```python
from build123d import *

# Parameters (mm, degrees)
ESQUISSE1_R             = 20
ESQUISSE1_R_2           = 8
BOSS_EXTRU_1_DEPTH      = 60
ESQUISSE2_W             = 40
ESQUISSE2_H             = 4.835178206
ESQUISSE2_W_2           = 44.689434038
ESQUISSE2_H_2           = 5.086258347
ENL_V_MAT_EXTRU_1_DEPTH = 60
TROU_TARAUD_M61_D       = 5
TROU_TARAUD_M61_DEPTH   = 13
TROU_TARAUD_M61_TIP     = 1.502151548
TROU_TARAUD_M62_D       = 5
TROU_TARAUD_M62_DEPTH   = 15
TROU_TARAUD_M62_TIP     = 1.502151548


with BuildPart() as part:
    # Esquisse1 → Boss.-Extru.1 (new body)
    with BuildSketch(Plane.XY):
        Circle(ESQUISSE1_R)
        Circle(ESQUISSE1_R_2, mode=Mode.SUBTRACT)
    extrude(amount=BOSS_EXTRU_1_DEPTH)

    # Esquisse2 → Enlèv. mat.-Extru.1 (cut)
    with BuildSketch(Plane.XY.offset(60)):
        with Locations((4.791370724, 19.417589103)):
            Rectangle(ESQUISSE2_W, ESQUISSE2_H)
        with Locations((-4.250423756, -19.543129173)):
            Rectangle(ESQUISSE2_W_2, ESQUISSE2_H_2)
    extrude(amount=-ENL_V_MAT_EXTRU_1_DEPTH, mode=Mode.SUBTRACT)

    # Trou taraudé M61
    with Locations(Plane(origin=(0, 17, 50), x_dir=(0, 0, 1), z_dir=(0, 1, 0))):
        with Locations((0, 0), (-40, 0)):
            Hole(TROU_TARAUD_M61_D / 2, depth=TROU_TARAUD_M61_DEPTH)
            with Locations((0, 0, -(TROU_TARAUD_M61_DEPTH + TROU_TARAUD_M61_TIP / 2))):  # 118° drill point
                Cone(0, TROU_TARAUD_M61_D / 2, TROU_TARAUD_M61_TIP, mode=Mode.SUBTRACT)

    # Trou taraudé M62
    with Locations(Plane(origin=(0, -17, 50), x_dir=(0, 0, -1), z_dir=(0, -1, 0))):
        with Locations((0, 0), (20, 0)):
            Hole(TROU_TARAUD_M62_D / 2, depth=TROU_TARAUD_M62_DEPTH)
            with Locations((0, 0, -(TROU_TARAUD_M62_DEPTH + TROU_TARAUD_M62_TIP / 2))):  # 118° drill point
                Cone(0, TROU_TARAUD_M62_D / 2, TROU_TARAUD_M62_TIP, mode=Mode.SUBTRACT)


solid = part.part
```
The listing builds one solid part. Answer for the finished solid, in the listing's coordinates (mm). A direction names the side the tool comes from. Coordinates: 2 decimals unless noted, no trailing zeros. Write each loop counter-clockwise with the first axis right and the second up, starting at its lowest first coordinate (ties: lowest second). Pieces come first, ordered by that corner, then holes. Notation, with made-up numbers: (61.5, -2) - (88.5, -2) arc R20 ccw to (88.5, 29) - close; hole circle Ø3 at (12.5, 29). An arc over 180 degrees is marked (long way). Return JSON: item names as keys, results as strings. Group by question number.
Q1. The part is cut by section A-A on z = 50. Write down the section's boundary in (x, y), and give its area (3 significant figures).
Q2. The part is cut by section B-B on z = 35. Write down the section's boundary in (x, y).
Q3. Find the intervals of material crossed by line 1 along Z through (x, y) = (0, 10.25); line 2 along Z through (x, y) = (0, -13.25); line 3 along Y through (x, z) = (0, 15), in increasing order. Write a range as [from, to].
Q4. The part is cut by section D-D on y = 3.5. Write down the section's boundary in (x, z).
Q5. Which of the six approach directions +Z, -Z, +X, -X, +Y, -Y give full straight-line access (tool end or side, diameter ignored) to faces 4 (the cylindrical face through (0.1, 12.2, 12.5)), 5 (the cylindrical face through (-0.96, 12.23, 47.69))?
Q6. For a pull along Y with two mould halves and no side action, classify faces 1 (the cylindrical face through (20, 0, 30)), 2 (the cylindrical face through (7.39, -3.06, 29.58)), 3 (the cylindrical face through (0.1, -12.2, 27.5)) as +Y half, -Y half, draft (parallel to the pull), parting line (faces both ways), or undercut.
Q7. Flat-ended cylindrical pins translate along their axes: pin 1 Ø4 at (x, z) = (0, 10) entering from +Y; pin 2 Ø12 at (y, z) = (13, 53.5) entering from +X (3 decimals); pin 3 Ø4 at (y, z) = (-8.5, 6.5) entering from -X. Find the tip coordinate at first contact, or state that the pin passes through.
Q8. The part is cut by section C-C on x = -1.5. Write down the section's boundary in (y, z), and give its area (3 significant figures).
Evaluation:
{
 "1": {"outline": "(-10.54, -17) - (-2.5, -17) - (-2.5, -7.6) arc R8 cw to (-2.5, 7.6) - (-2.5, 17) - (-10.54, 17) arc R20 ccw to start; (2.5, -17) - (10.54, -17) arc R20 ccw to (10.54, 17) - (2.5, 17) - (2.5, 7.6) arc R8 cw to (2.5, -7.6) - close", "area": "879 mm2"},
 "2": {"outline": "(-10.54, -17) - (10.54, -17) arc R20 ccw to (10.54, 17) - (-10.54, 17) arc R20 ccw to start; hole circle Ø16 at (0, 0)"},
 "3": {"line 1": "z = [0, 7.5], [12.5, 47.5], [52.5, 60]", "line 2": "z = [0, 27.5], [32.5, 47.5], [52.5, 60]", "line 3": "y = [-17, -8], [8, 17]"},
 "4": {"outline": "(-19.69, 0) - (-7.19, 0) - (-7.19, 60) - (-19.69, 60) - close; (7.19, 0) - (19.69, 0) - (19.69, 60) - (7.19, 60) - close"},
 "5": {"face 4": "+Y", "face 5": "+Y, -Y"},
 "6": {"face 1": "parting line", "face 2": "undercut", "face 3": "draft"},
 "7": {"pin 1": "stops at y = -7.75", "pin 2": "stops at x = 18.735", "pin 3": "stops at x = -18.91"},
 "8": {"outline": "(-17, 0) - (-7.86, 0) - (-7.86, 28) - (-17, 28) - close; (-17, 32) - (-7.86, 32) - (-7.86, 48) - (-17, 48) - close; (-17, 52) - (-7.86, 52) - (-7.86, 60) - (-17, 60) - close; (7.86, 0) - (17, 0) - (17, 8) - (7.86, 8) - close; (7.86, 12) - (17, 12) - (17, 48) - (7.86, 48) - close; (7.86, 52) - (17, 52) - (17, 60) - (7.86, 60) - close", "area": "951 mm2"}
}
